Part model, mm, in its own coordinate system. A direction names the side the tool comes from. Give positions to 0.01 mm unless a question says otherwise; leave off trailing zeros. Write each loop counter-clockwise with the first axis right and the second up, starting at its lowest first coordinate (ties: lowest second). Pieces come first, ordered by that corner, then holes. Notation, with made-up numbers: M 62.5,29 L 113.5,29 A20 ccw 113.5,63 Z; hole C -25.5,0 d8. An arc over 180 degrees is marked long. Answer as CSV lines item,"result". Start each with the question number.
1) Slice it at D-D, the plane z = 6. Give the cut face in (x, y).
2) Mould opens along Z. For faces 6 (the cylindrical face through (-0.108, 0.848, 0.662)), 7 (the flat face through (12.829, -2.518, 6.371)), 8 (the flat face through (0, 11.902, 2)) say: pulls with the +Z half, pulls with the -Z half, needs draft (parallel to the pull), parting line crosses it, or undercut.
3) Slice it at A-A, the plane z = 1.15. Give the cut face in (x, y), plus the area to 3 significant figures.
4) Wall check: line 1 along Y through (x, z) = (-2, 3.5); line 2 along Z through (x, y) = (4, -6.5); line 3 along Y through (x, z) = (12.8, 0.75). Give the ranges that are in metal, low to high. Write a range as from..to.
5) Slice it at B-B, the plane y = -1.5. Give the cut face in (x, z).
6) Tool access for faces 1 (the cylindrical face through (-12.323, 0.05, 0.796)), 2 (the flat face through (14.9, 0, 6)), 3 (the flat face through (12.1, 13.48, 1.35)), 4 (the cylindrical face through (-8.8, -10.5, 1.4)), 5 (the flat face through (-21, 0, 2)): list every direction of +Z, -Z, +X, -X, +Y, -Y with a clear straight run to the whole face (end or side of a thin tool).
7) Pin check, flat tips, straight feed: pin 1 Ø1.6 at (x, y) = (21, 5) entering from +Z; pin 2 Ø2 at (x, z) = (1.5, 4) entering from -Y; pin 3 Ø5.5 at (x, z) = (1.5, 0) entering from +Y; pin 4 Ø1 at (x, z) = (-0.5, 6.5) entering from -Y. Stop position of each tip, or through.
8) Slice it at C-C, the plane x = 0. Give the cut face in (y, z), plus the area to 3 significant figures.
```python
from build123d import *

# Parameters (mm, degrees)
SKETCH_W        = 44
SKETCH_H        = 42
PAD_DEPTH       = 2
SKETCH001_W     = 40
SKETCH001_H     = 42
PAD001_DEPTH    = 2.85
SKETCH002_W     = 4.2
SKETCH002_H     = 5.6
PAD002_DEPTH    = 3
POCKET_DEPTH    = 44.001
SKETCH004_W     = 40
SKETCH004_H     = 8.35
PAD003_DEPTH    = 15
SKETCH005_W     = 40
SKETCH005_H     = 8.35
PAD004_DEPTH    = 15
POCKET001_DEPTH = 42.001
POCKET002_DEPTH = 13.201
FILLET_R        = 0.4
SKETCH008_W     = 44
SKETCH008_H     = 2.55
PAD005_DEPTH    = 42
POCKET003_DEPTH = 2.551
SKETCH009_R     = 0.5
POCKET004_DEPTH = 42.001
POCKET010_DEPTH = 17.851
CHAMFER002_SIZE = 0.5
POCKET017_START = -0.8
SKETCH019_R     = 0.5
POCKET017_DEPTH = 24.2


with BuildPart() as part:
    # Sketch → Pad (new body)
    with BuildSketch(Plane.XY):
        Rectangle(SKETCH_W, SKETCH_H)
    extrude(amount=PAD_DEPTH)

    # Sketch001 (on Face6 of Pad) → Pad001 (join)
    with BuildSketch(Plane.XY.offset(2)):
        Rectangle(SKETCH001_W, SKETCH001_H)
    extrude(amount=PAD001_DEPTH)

    # Sketch002 (on Face8 of Pad001) → Pad002 (join)
    with BuildSketch(Plane.XY.offset(4.85)):
        with Locations((-12.8, -0.1)):
            Rectangle(SKETCH002_W, SKETCH002_H)
        with Locations((12.8, -0.1)):
            Rectangle(SKETCH002_W, SKETCH002_H)
    extrude(amount=PAD002_DEPTH)

    # Sketch003 (on Face1 of Pad002) → Pocket (cut, through all)
    with BuildSketch(Plane.YZ.offset(22)):
        Polygon((-2.9, 4.85), (-2.9, 8.35), (-2.02, 8.35), align=None)
        Polygon((2.7, 8.35), (2.7, 4.85), (1.82, 8.35), align=None)
    extrude(amount=-POCKET_DEPTH, mode=Mode.SUBTRACT)

    # Sketch004 (on Face2 of Pocket) → Pad003 (join)
    with BuildSketch(Plane.XZ.offset(21)):
        with Locations((0, 9.025)):
            Rectangle(SKETCH004_W, SKETCH004_H)
    extrude(amount=-PAD003_DEPTH)

    # Sketch005 (on Face2 of Pad003) → Pad004 (join)
    with BuildSketch(Plane(origin=(0, 21, 0), x_dir=(-1, 0, 0), z_dir=(0, 1, 0))):
        with Locations((0, 9.025)):
            Rectangle(SKETCH005_W, SKETCH005_H)
    extrude(amount=-PAD004_DEPTH)

    # Sketch006 (on Face24 of Pad004) → Pocket001 (cut, through all)
    with BuildSketch(Plane(origin=(-20, 0, 0), x_dir=(0, -1, 0), z_dir=(-1, 0, 0))):
        with BuildLine():
            Line((-21, 13.2), (-20, 13.2))
            ThreePointArc((-20, 13.2), (-20.707107, 12.907107), (-21, 12.2))
            Line((-21, 12.2), (-21, 13.2))
        make_face()
        with BuildLine():
            ThreePointArc((-15, 12.2), (-15.292893, 12.907107), (-16, 13.2))
            Line((-16, 13.2), (-6, 13.2))
            Line((-6, 13.2), (-6, 4.85))
            Line((-6, 4.85), (-18.25, 4.85))
            Line((-18.25, 10.6), (-18.25, 4.85))
            Line((-17.125, 10.6), (-18.25, 10.6))
            ThreePointArc((-17.125, 10.6), (-15.794998, 11.044723), (-15, 12.2))
        make_face()
        with BuildLine():
            Line((18.35, 4.85), (18.35, 11.2))
            Line((18.35, 11.2), (16, 11.2))
            ThreePointArc((16, 13.2), (15, 12.2), (16, 11.2))
            Line((6, 13.2), (16, 13.2))
            Line((6, 4.85), (6, 13.2))
            Line((6, 4.85), (18.35, 4.85))
        make_face()
    extrude(amount=-POCKET001_DEPTH, mode=Mode.SUBTRACT)

    # Sketch007 (on Face18 of Pocket001) → Pocket002 (cut, through all)
    with BuildSketch(Plane(origin=(0, 0, 0), x_dir=(1, 0, 0), z_dir=(0, 0, -1))):
        with BuildLine():
            ThreePointArc((-17, 21), (-20.535534, 19.535534), (-22, 16))
            Line((-22, 21), (-22, 16))
            Line((-17, 21), (-22, 21))
        make_face()
        with BuildLine():
            ThreePointArc((22, 16), (20.535534, 19.535534), (17, 21))
            Line((22, 21), (17, 21))
            Line((22, 16), (22, 21))
        make_face()
        with BuildLine():
            ThreePointArc((17, -21), (20.535534, -19.535534), (22, -16))
            Line((22, -21), (22, -16))
            Line((22, -21), (17, -21))
        make_face()
        with BuildLine():
            ThreePointArc((-22, -16), (-20.535534, -19.535534), (-17, -21))
            Line((-22, -21), (-17, -21))
            Line((-22, -16), (-22, -21))
        make_face()
    extrude(amount=-POCKET002_DEPTH, mode=Mode.SUBTRACT)

    # Fillet
    fillet_edges = [part.edges().sort_by_distance(p)[0] for p in [
        (0, -21, 13.2),
        (20, -18, 13.2),
        (-20, -18, 13.2),
        (20, -18.35, 8.025),
        (-20, -18.35, 8.025),
        (-20, 18, 13.2),
        (20, 18, 13.2),
        (20, 17.6875, 10.6),
        (20, 18.25, 7.725),
        (-20, 18.25, 7.725),
        (-20, 17.6875, 10.6),
        (20, -0.05, 4.85),
        (-20, -0.05, 4.85),
    ]]
    fillet(fillet_edges, radius=FILLET_R)

    # Sketch008 (on Face15 of Clone) → Pad005 (new body)
    with BuildSketch(Plane.XZ.offset(21)):
        with Locations((0, -1.275)):
            Rectangle(SKETCH008_W, SKETCH008_H)
    extrude(amount=-PAD005_DEPTH)

    # ShapeBinder → Pocket003 (cut, through all)
    with BuildSketch(Plane(origin=(-20.88316, 19.88316, 0), x_dir=(0, 1, 0), z_dir=(0, 0, 1))):
        with BuildLine():
            Line((1.11684, 1.11684), (-3.88316, 1.11684))
            ThreePointArc((-3.88316, 1.11684), (-0.347626, -0.347626), (1.11684, -3.88316))
            Line((1.11684, -3.88316), (1.11684, 1.11684))
        make_face()
        with BuildLine():
            Line((-40.88316, 1.11684), (-40.88316, -3.88316))
            ThreePointArc((-40.88316, -3.88316), (-39.418694, -0.347626), (-35.88316, 1.11684))
            Line((-35.88316, 1.11684), (-40.88316, 1.11684))
        make_face()
        with BuildLine():
            Line((-40.88316, -37.88316), (-40.88316, -42.88316))
            Line((-40.88316, -42.88316), (-35.88316, -42.88316))
            ThreePointArc((-35.88316, -42.88316), (-39.418694, -41.418694), (-40.88316, -37.88316))
        make_face()
        with BuildLine():
            ThreePointArc((1.11684, -37.88316), (-0.347626, -41.418694), (-3.88316, -42.88316))
            Line((-3.88316, -42.88316), (1.11684, -42.88316))
            Line((1.11684, -42.88316), (1.11684, -37.88316))
        make_face()
    extrude(amount=-POCKET003_DEPTH, mode=Mode.SUBTRACT)

    # Sketch009 (on Face29 of Pocket003) → Pocket004 (cut, through all)
    with BuildSketch(Plane.XZ.offset(21)):
        with Locations((0, 1.15)):
            Circle(SKETCH009_R)
    extrude(amount=-POCKET004_DEPTH, mode=Mode.SUBTRACT)

    # ShapeBinder005 → Pocket010 (cut, through all)
    with BuildSketch(Plane(origin=(0, -16.15872, -4.65), x_dir=(0, 1, 0), z_dir=(0, 0, 1))):
        with BuildLine():
            Line((1.45872, -22), (1.45872, -20.8))
            ThreePointArc((1.45872, -20.8), (2.067221, -16.604371), (3.842579, -12.754477))
            ThreePointArc((3.842579, -12.754477), (5.641979, -8.852447), (6.25872, -4.6))
            Line((6.25872, -4.6), (6.25872, 4.6))
            ThreePointArc((6.25872, 4.6), (5.641979, 8.852447), (3.842579, 12.754477))
            ThreePointArc((3.842579, 12.754477), (2.067221, 16.60437), (1.45872, 20.8))
            Line((1.45872, 20.8), (1.45872, 22))
            Line((1.45872, 22), (0.15872, 22))
            ThreePointArc((0.15872, 22), (-3.376814, 20.535534), (-4.84128, 17))
            Line((-4.84128, 17), (-4.84128, -17))
            ThreePointArc((-4.84128, -17), (-3.376814, -20.535534), (0.15872, -22))
            Line((0.15872, -22), (1.45872, -22))
        make_face()
        with BuildLine():
            Line((37.15872, -17), (37.15872, 17))
            ThreePointArc((37.15872, 17), (35.694254, 20.535534), (32.15872, 22))
            Line((32.15872, 22), (31.260407, 22))
            Line((31.260407, 22), (31.260407, 20.818291))
            Line((31.260407, 20.818291), (28.060407, 3.618291))
            Line((28.060407, 3.618291), (28.060407, -3.618291))
            Line((28.060407, -3.618291), (31.260407, -20.818291))
            Line((31.260407, -20.818291), (31.260407, -22))
            Line((31.260407, -22), (32.15872, -22))
            ThreePointArc((32.15872, -22), (35.694254, -20.535534), (37.15872, -17))
        make_face()
    extrude(amount=POCKET010_DEPTH, mode=Mode.SUBTRACT)

    # Chamfer002
    chamfer002_edges = [part.edges().sort_by_distance(p)[0] for p in [
        (-21.4, -14.7, -2.55),
        (-16.604371, -14.0915, -2.55),
        (-8.852447, -10.516741, -2.55),
        (0, -9.9, -2.55),
        (8.852447, -10.516741, -2.55),
        (16.604371, -14.0915, -2.55),
        (21.4, -14.7, -2.55),
        (22, 0.200843, -2.55),
        (21.409145, 15.101687, -2.55),
        (12.218291, 13.501687, -2.55),
        (0, 11.901687, -2.55),
        (-12.218291, 13.501687, -2.55),
        (-21.409145, 15.101687, -2.55),
        (-22, 0.200843, -2.55),
        (22, 15.101687, -0.275),
        (22, -14.7, -0.275),
        (-22, -14.7, -0.275),
        (-22, 15.101687, -0.275),
    ]]
    chamfer(chamfer002_edges, length=CHAMFER002_SIZE)

    # Sketch019 → Pocket017 (cut)
    with BuildSketch(Plane.XY.offset(4.85).offset(POCKET017_START)):
        with Locations((-12.8, -0.1)):
            Circle(SKETCH019_R)
        with Locations((12.8, -0.1)):
            Circle(SKETCH019_R)
    extrude(amount=-POCKET017_DEPTH, mode=Mode.SUBTRACT)


solid = part.part
```
Found:
1,outline,"M -14.9,-2.61 L -10.7,-2.61 L -10.7,2.41 L -14.9,2.41 Z; M 10.7,-2.61 L 14.9,-2.61 L 14.9,2.41 L 10.7,2.41 Z"
2,face 6,"undercut"
2,face 7,"pulls with the +Z half"
2,face 8,"needs draft"
3,outline,"M -22,-14.2 L -21.5,-14.7 L -20.8,-14.7 A14.77 ccw -12.75,-12.32 A14.97 cw -4.6,-9.9 L -0.5,-9.9 L -0.5,11.9 L -3.62,11.9 L -20.82,15.1 L -21.5,15.1 L -22,14.6 Z; M 0.5,-9.9 L 4.6,-9.9 A14.97 cw 12.75,-12.32 A14.77 ccw 20.8,-14.7 L 21.5,-14.7 L 22,-14.2 L 22,14.6 L 21.5,15.1 L 20.82,15.1 L 3.62,11.9 L 0.5,11.9 Z; hole C -12.8,-0.1 d1; hole C 12.8,-0.1 d1"
3,area,"1,090 mm²"
4,line 1,"-9.9..11.9"
4,line 2,"-2.55..4.85"
4,line 3,"-12.35..-0.6, 0.4..13.61"
5,outline,"M -22,-2.05 L -21.5,-2.55 L 21.5,-2.55 L 22,-2.05 L 22,2 L 20,2 L 20,4.45 A0.4 ccw 19.6,4.85 L 14.9,4.85 L 14.9,7.85 L 10.7,7.85 L 10.7,4.85 L -10.7,4.85 L -10.7,7.85 L -14.9,7.85 L -14.9,4.85 L -19.6,4.85 A0.4 ccw -20,4.45 L -20,2 L -22,2 Z; hole C 0,1.15 d1"
6,face 1,"-Z"
6,face 2,"+Z, +X, +Y, -Y"
6,face 3,"+Z, -Z, +Y"
6,face 4,"+Z, -Z, -Y"
6,face 5,"+Z, -X, +Y, -Y"
7,pin 1,"z = 2"
7,pin 2,"y = -9.9"
7,pin 3,"y = 12.02"
7,pin 4,"through"
8,outline,"M -9.9,-2.05 L -9.4,-2.55 L 11.4,-2.55 L 11.9,-2.05 L 11.9,0.65 L -9.9,0.65 Z; M -9.9,1.65 L 11.9,1.65 L 11.9,4.85 L -9.9,4.85 Z"
8,area,"139 mm²"
